For this review, take the finished solid that the model builds, in its own axes (mm). A direction names the side the tool comes from. Round coordinates to 2 decimals unless told otherwise and drop trailing zeros. Write each loop counter-clockwise with the first axis right and the second up, starting at its lowest first coordinate (ties: lowest second). Pieces come first, ordered by that corner, then holes. Notation, with made-up numbers: M 85.25,-21 L 136.25,-21 A33 cw 136.25,15 Z; hole C 86.25,89 d8. An arc over 180 degrees is marked long. Use one line per item in the form item = value. Start each with the question number.
Item 1: For faces 4 (the cylindrical face through (-3.905, 2.465, 0.867)), 5 (the cylindrical face through (-4.596, 19.474, 11.085)), 6 (the cylindrical face through (-3.955, 58.311, -5.158)), 7 (the flat face through (0, 75, 0)), 8 (the flat face through (11, 35, 0)), list the 3-axis set-ups (+Z, -Z, +X, -X, +Y, -Y) from which the entire face can be reached by the end or side of a thin tool; tool diameter is ignored.
Item 2: For line 1 (X direction, y = 2.65, z = 0); line 2 (Y direction, x = 2.5, z = 2.25); line 3 (Y direction, x = 10.5, z = -4.5), list the stretches that pass through material, from the lowest coordinate up. Write a range as [from, to].
Item 3: Draft analysis for pull direction X (two halves, no side actions). For faces 1 (the flat face through (3, 0, -3)), 2 (the flat face through (0, 5, 0)), 3 (the flat face through (-11, 35, 0)), state which applies: released by +X, released by -X, zero draft, split by the parting line, or undercut.
Item 4: For P1, Ø0.8, axis at x = 11.5, z = 2, coming from the +Y side; P2, Ø4, axis at y = 28.5, z = 8.5, coming from the +X side; P3, Ø4, axis at x = -1, y = 47.5, coming from the +Z side, all flat-tipped, find the tip position at first contact; note any pin that passes through.
Item 5: Add section B-B (y = 15). State the section outline as (x, z) points, and give its area (3 significant figures).
Item 6: Add section C-C (y = 68.5). State the section outline as (x, z) points.
Item 7: Add section A-A (z = 0). State the section outline as (x, y) points, and give its area (3 significant figures).
from build123d import *

# Parameters (mm, degrees)
SKETCH1_R               = 12
BOSS_EXTRUDE1_DEPTH     = 40
SKETCH2_R               = 6.5
BOSS_EXTRUDE2_DEPTH     = 35
FILLET1_R               = 3
FILLET2_R               = 5
FILLET3_R               = 0.5
CUT_EXTRUDE1_DEPTH      = 77.896033821
CUT_EXTRUDE1_DEPTH_BACK = 77.896033821
SKETCH3_W               = 1
SKETCH3_H               = 10
SKETCH4_R               = 4
CUT_EXTRUDE2_DEPTH      = 5


with BuildPart() as part:
    # Sketch1 → Boss-Extrude1 (new body)
    with BuildSketch(Plane(origin=(0, 0, 0), x_dir=(1, 0, 0), z_dir=(0, 1, 0))):
        with Locations(Location((0, 0, 0), (0, 0, 270))):
            Circle(SKETCH1_R)
    extrude(amount=BOSS_EXTRUDE1_DEPTH)

    # Sketch2 → Boss-Extrude2 (add)
    with BuildSketch(Plane(origin=(0, 40, 0), x_dir=(1, 0, 0), z_dir=(0, 1, 0))):
        with Locations(Location((0, 0, 0), (0, 0, 270))):
            Circle(SKETCH2_R)
    extrude(amount=BOSS_EXTRUDE2_DEPTH)

    # Fillet1
    fillet1_edges = [part.edges().sort_by_distance(p)[0] for p in [
        (0, 75, -6.5),
    ]]
    fillet(fillet1_edges, radius=FILLET1_R)

    # Fillet2
    fillet2_edges = [part.edges().sort_by_distance(p)[0] for p in [
        (0, 40, -6.5),
    ]]
    fillet(fillet2_edges, radius=FILLET2_R)

    # Fillet3
    fillet3_edges = [part.edges().sort_by_distance(p)[0] for p in [
        (0, 40, -12),
    ]]
    fillet(fillet3_edges, radius=FILLET3_R - 0.0001)  # a hair under: the kernel refuses the full size

    # Sketch3 → Cut-Extrude1 (cut, two sides: drawn at the far end of the back side and taken through both)
    with BuildSketch(Plane.XY.offset(-CUT_EXTRUDE1_DEPTH_BACK)):
        with Locations((-11.5, 35.09742525)):
            Rectangle(SKETCH3_W, SKETCH3_H)
        with Locations((11.5, 35.09742525)):
            Rectangle(SKETCH3_W, SKETCH3_H)
    extrude(amount=CUT_EXTRUDE1_DEPTH + CUT_EXTRUDE1_DEPTH_BACK, mode=Mode.SUBTRACT)

    # Sketch4 → Cut-Extrude2 (cut)
    with BuildSketch(Plane.XZ):
        with Locations(Location((0, 0, 0), (0, 0, 270))):
            Circle(SKETCH4_R)
    extrude(amount=-CUT_EXTRUDE2_DEPTH, mode=Mode.SUBTRACT)


solid = part.part
Calculated:
q1.face_4 = -Y
q1.face_5 = +Y, -Y
q1.face_6 = +Y
q1.face_7 = +Z, -Z, +X, -X, +Y
q1.face_8 = +Z, -Z, +X, +Y
q2.line_1 = [-12, -4], [4, 12]
q2.line_2 = [5, 75]
q2.line_3 = [0, 40]
q3.face_1 = zero draft
q3.face_2 = undercut
q3.face_3 = released by -X
q4.P1 = 30.1
q4.P2 = 10.09
q4.P3 = 6.5
q5.outline = C 0,0 d24
q5.area = 452 mm^2
q6.outline = C 0,0 d13
q7.outline = M -12,0 L -4,0 L -4,5 L 4,5 L 4,0 L 12,0 L 12,30.1 L 11,30.1 L 11,40.03 A5 cw 6.5,45 L 6.5,72 A3 ccw 3.5,75 L -3.5,75 A3 ccw -6.5,72 L -6.5,45 A5 cw -11,40.03 L -11,30.1 L -12,30.1 Z
q7.area = 1,360 mm^2
